For this review, take the finished solid that the model builds, in its own axes (mm). Face numbers are marked on the shaded views. A direction names the side the tool comes from. Give positions to 0.01 mm unless a question says otherwise; leave off trailing zeros. Write each loop counter-clockwise with the first axis right and the second up, starting at its lowest first coordinate (ties: lowest second). Pieces come first, ordered by that corner, then holes. Notation, with made-up numbers: M 35.25,72.25 L 61.25,72.25 A12 cw 61.25,92.25 Z; hole C -12,65.25 d9. An arc over 180 degrees is marked long. One line per item, written item: value. Start each with the question number.
Item 1: Consider section B-B, the plane x = 24.5. Write out the cut boundary in (y, z), and give its area (3 significant figures).
Item 2: Clearance check with flat-ended pins moving along their axes: pin 1 Ø2 at (x, y) = (-9, -72) entering from +Z; pin 2 Ø20 at (x, z) = (24.5, 5) entering from -Y; pin 3 Ø6 at (x, y) = (3.5, -60.5) entering from +Z; pin 4 Ø4 at (x, y) = (8, -188.5) entering from -Z. State where each tip first meets the part, or that it passes through.
Item 3: To check wall thickness, follow probe 1 along X at (y, z) = (-223.5, 5); probe 2 along Z at (x, y) = (24.5, -130); probe 3 along Z at (x, y) = (-73, -70). State the ranges of each line that lie inside material, in increasing order.
Item 4: Consider section C-C, the plane y = -97. Write out the cut boundary in (x, z).
Item 5: Consider section A-A, the plane z = 5. Write out the cut boundary in (x, y), and give its area (3 significant figures).
Item 6: Mouldability with a two-part tool opening along X and no side actions: class the marked faces 1, 2 and 3 as released by +X, released by -X, zero draft, split by the parting line, or undercut.
Item 7: Tool access review of the marked faces 4 and 5: name each direction out of +Z, -Z, +X, -X, +Y, -Y from which nothing blocks a thin tool from reaching the whole face with its end or side.
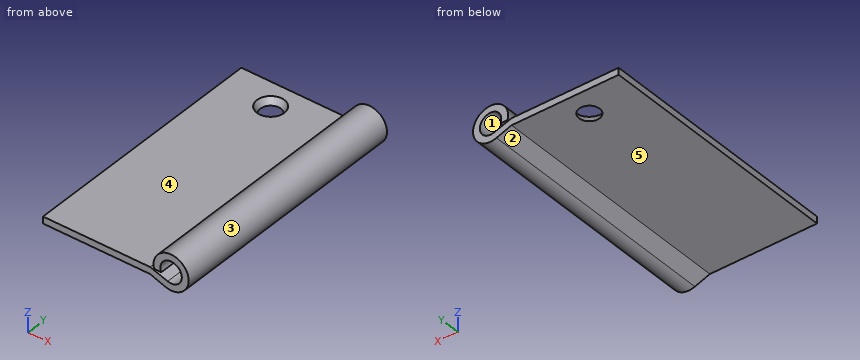
```python
from build123d import *

# Parameters (mm, degrees)
F1_DEPTH = 292
F3_R     = 12
F2_R     = 16


with BuildPart() as f1:
    # F0 (on Front) → F1 (new body)
    with BuildSketch(Plane.XZ):
        with BuildLine():
            Line((20.542224, -6.856897), (0, 0))
            Line((0, 0), (-125, 0))
            Line((-125, 0), (-125, -8))
            Line((-125, -8), (0, -8))
            Line((0, -8), (17.58743, -14.299388))
            ThreePointArc((17.58743, -14.299388), (39.685209, 18.77169), (4.619105, 0))
            Line((4.619105, 0), (13.043561, 0))
            ThreePointArc((13.043561, 0), (32.935269, 14.224762), (20.542224, -6.856897))
        make_face()
    extrude(amount=F1_DEPTH)

    # F3 (on face) → F4 section 0
    with BuildSketch(Plane(origin=(0, 0, -8), x_dir=(1, 0, 0), z_dir=(0, 0, -1))):
        with Locations((-67, 30)):
            Circle(F3_R)
    # F2 (on face) → F4 section 1
    with BuildSketch(Plane.XY):
        with Locations((-67, -30)):
            Circle(F2_R)
    loft(mode=Mode.SUBTRACT)


solid = f1.part
```
Model answer:
1. outline: M -292,-15.5 L 0,-15.5 L 0,-7.5 L -292,-7.5 Z; M -292,17.5 L 0,17.5 L 0,25.5 L -292,25.5 Z
1. area: 4,670 mm2
2. pin 1: stops at z = 0
2. pin 2: passes through
2. pin 3: stops at z = 14.81
2. pin 4: stops at z = -11.58
3. probe 1: x = 4 to 12, 37 to 45
3. probe 2: z = -15.5 to -7.5, 17.5 to 25.5
3. probe 3: z = -8 to 0
4. outline: M -125,-8 L 0,-8 L 17.59,-14.3 A20.5 ccw long 4.62,0 L 13.04,0 A12.5 cw long 20.54,-6.86 L 0,0 L -125,0 Z
5. outline: M 4,-292 L 12,-292 L 12,0 L 4,0 Z; M 37,-292 L 45,-292 L 45,0 L 37,0 Z
5. area: 4,670 mm2
6. face 1: undercut
6. face 2: released by -X
6. face 3: split by the parting line
7. face 4: +Z, -X, +Y, -Y
7. face 5: -Z, -X, +Y, -Y
